CAD build for the part. Positions are in the model's coordinates, mm. A direction names the side the tool comes from. Give positions to 0.01 mm unless a question says otherwise; leave off trailing zeros. Write each loop counter-clockwise with the first axis right and the second up, starting at its lowest first coordinate (ties: lowest second). Pieces come first, ordered by that corner, then holes. Notation, with made-up numbers: (-17.5, 59) -> (-13.5, 59) arc R31 ccw to (-13.5, 86) -> close; hole circle Ø4 at (70, 3). An arc over 180 degrees is marked (long way). Answer as a JSON object with one key per item and string values.
```python
from build123d import *

# Parameters (mm, degrees)
SKETCH002_R                 = 3
EXTRUDE002_DEPTH            = 4
EXTRUDE002_DEPTH_BACK       = 3.4
CYLINDER049_R               = 1.5
CYLINDER049_DEPTH           = 19
CYLINDER014_R               = 2
CYLINDER014_DEPTH           = 1
CYLINDER014_PLACEMENT_ANGLE = 45
CYLINDER015_R               = 2
CYLINDER015_DEPTH           = 1
CYLINDER016_R               = 2
CYLINDER016_DEPTH           = 1
CYLINDER016_PLACEMENT_ANGLE = 135
CYLINDER017_R               = 2
CYLINDER017_DEPTH           = 1
CYLINDER018_R               = 2
CYLINDER018_DEPTH           = 5
CYLINDER018_PLACEMENT_ANGLE = 225
CYLINDER019_R               = 2
CYLINDER019_DEPTH           = 5
CYLINDER020_R               = 2
CYLINDER020_DEPTH           = 5
CYLINDER020_PLACEMENT_ANGLE = 45
CYLINDER013_R               = 2
CYLINDER013_DEPTH           = 1
CYLINDER021_R               = 5
CYLINDER021_DEPTH           = 5
CYLINDER012_R               = 25
CYLINDER012_DEPTH           = 1.5
CUT050_PLACEMENT_ANGLE      = 180


with BuildPart() as extrude002:
    # Sketch002 (on Face25 of Shape005) → Extrude002 (new body, two sides)
    with BuildSketch(Plane(origin=(85.664098, -4.553146, 1.091283), x_dir=(-1, 0, 0), z_dir=(0, 0, 1))) as extrude002_sk:
        with Locations((9.450198, -0.000218)):
            Circle(SKETCH002_R)
    extrude(amount=EXTRUDE002_DEPTH)
    extrude(extrude002_sk.sketch, amount=-EXTRUDE002_DEPTH_BACK)


with BuildPart() as extrude002_1:
    # Extrude002 placement: moved
    add(extrude002.part.moved(Location((-76.21, 4.55, 3))))


with BuildPart() as cylinder049:
    # Cylinder049 → Cylinder049 (new body)
    with BuildSketch(Plane.XY.offset(-1)):
        Circle(CYLINDER049_R)
    extrude(amount=CYLINDER049_DEPTH)


with BuildPart() as cylinder014:
    # cylinder014 → cylinder014 (new body)
    with BuildSketch(Plane.XY):
        Circle(CYLINDER014_R)
    extrude(amount=CYLINDER014_DEPTH)


with BuildPart() as cylinder014_1:
    # cylinder014 placement: moved
    add(cylinder014.part.moved(Location((13.081475, 13.081475, 0))).rotate(Axis((13.081475, 13.081475, 0), (0, 0, 1)), CYLINDER014_PLACEMENT_ANGLE))


with BuildPart() as cylinder015:
    # cylinder015 → cylinder015 (new body)
    with BuildSketch(Plane(origin=(0, 18.5, 0), x_dir=(0, 1, 0), z_dir=(0, 0, 1))):
        Circle(CYLINDER015_R)
    extrude(amount=CYLINDER015_DEPTH)


with BuildPart() as cylinder016:
    # cylinder016 → cylinder016 (new body)
    with BuildSketch(Plane.XY):
        Circle(CYLINDER016_R)
    extrude(amount=CYLINDER016_DEPTH)


with BuildPart() as cylinder016_1:
    # cylinder016 placement: moved
    add(cylinder016.part.moved(Location((-13.081475, 13.081475, 0))).rotate(Axis((-13.081475, 13.081475, 0), (0, 0, 1)), CYLINDER016_PLACEMENT_ANGLE))


with BuildPart() as cylinder017:
    # cylinder017 → cylinder017 (new body)
    with BuildSketch(Plane(origin=(-18.5, 0, 0), x_dir=(-1, 0, 0), z_dir=(0, 0, 1))):
        Circle(CYLINDER017_R)
    extrude(amount=CYLINDER017_DEPTH)


with BuildPart() as cylinder018:
    # cylinder018 → cylinder018 (new body)
    with BuildSketch(Plane.XY):
        Circle(CYLINDER018_R)
    extrude(amount=CYLINDER018_DEPTH)


with BuildPart() as cylinder018_1:
    # cylinder018 placement: moved
    add(cylinder018.part.moved(Location((-13.081475, -13.081475, 0))).rotate(Axis((-13.081475, -13.081475, 0), (0, 0, 1)), CYLINDER018_PLACEMENT_ANGLE))


with BuildPart() as cylinder019:
    # cylinder019 → cylinder019 (new body)
    with BuildSketch(Plane(origin=(0, -18.5, 0), x_dir=(0, -1, 0), z_dir=(0, 0, 1))):
        Circle(CYLINDER019_R)
    extrude(amount=CYLINDER019_DEPTH)


with BuildPart() as cylinder020:
    # cylinder020 → cylinder020 (new body)
    with BuildSketch(Plane.XY):
        Circle(CYLINDER020_R)
    extrude(amount=CYLINDER020_DEPTH)


with BuildPart() as cylinder020_1:
    # cylinder020 placement: moved
    add(cylinder020.part.moved(Location((13.081475, -13.081475, 0))).rotate(Axis((13.081475, -13.081475, 0), (0, 0, -1)), CYLINDER020_PLACEMENT_ANGLE))


with BuildPart() as fusion026:
    # cylinder013 → cylinder013 (new body)
    with BuildSketch(Plane(origin=(18.5, 0, 0), x_dir=(1, 0, 0), z_dir=(0, 0, 1))):
        Circle(CYLINDER013_R)
    extrude(amount=CYLINDER013_DEPTH)

    # Group001: union cylinder014, cylinder015, cylinder016, cylinder017, cylinder018, cylinder019, cylinder020
    add(cylinder014_1.part)
    add(cylinder015.part)
    add(cylinder016_1.part)
    add(cylinder017.part)
    add(cylinder018_1.part)
    add(cylinder019.part)
    add(cylinder020_1.part)


with BuildPart() as fusion026_1:
    # Group001 placement: moved
    add(fusion026.part.moved(Location((0, 0, -1))))

    # Fusion026: union Extrude002, Cylinder049
    add(extrude002_1.part)
    add(cylinder049.part)


with BuildPart() as servo_central_shaft002:
    # cylinder021 → cylinder021 (new body)
    with BuildSketch(Plane.XY):
        Circle(CYLINDER021_R)
    extrude(amount=CYLINDER021_DEPTH)


with BuildPart() as rotor:
    # cylinder012 → cylinder012 (new body)
    with BuildSketch(Plane.XY):
        Circle(CYLINDER012_R)
    extrude(amount=CYLINDER012_DEPTH)

    # Fusion027: union servo_central_shaft002
    add(servo_central_shaft002.part)

    # Cut050: cut Fusion026
    add(fusion026_1.part, mode=Mode.SUBTRACT)


with BuildPart() as rotor_1:
    # Cut050 placement: moved
    add(rotor.part.moved(Location((-13.7, 55.5, 5))).rotate(Axis((-13.7, 55.5, 5), (1, 0, 0)), CUT050_PLACEMENT_ANGLE))


solid = rotor_1.part
```
1) Mould opens along X. For faces 3 (the cylindrical face through (-14.351, 50.543, 1.775)), 4 (the flat face through (-10, 55, 0)), 5 (the cylindrical face through (0.15, 70.43, 4.26)) say: released by +X, released by -X, zero draft, split by the parting line, or undercut.
Model answer:
{"face 3": "split by the parting line", "face 4": "zero draft", "face 5": "undercut"}
2) Slice it at B-B (y = 73). List the corners of the cut face in (x, z).
Model answer:
{"outline": "(-31.55, 3.5) -> (-15.43, 3.5) -> (-15.43, 5) -> (-31.55, 5) -> close; (-11.97, 3.5) -> (4.15, 3.5) -> (4.15, 5) -> (-11.97, 5) -> close"}
3) Slice it at C-C (x = -26.5). List the corners of the cut face in (y, z).
Model answer:
{"outline": "(34.03, 3.5) -> (66.6, 3.5) -> (66.6, 5) -> (34.03, 5) -> close; (70.56, 3.5) -> (76.97, 3.5) -> (76.97, 5) -> (70.56, 5) -> close"}
4) Wall check: probe 1 along Y at (x, z) = (-13.7, 4.15); probe 2 along Z at (x, y) = (0, 42); probe 3 along Y at (x, z) = (-1, 3.9). Give the ranges that are in metal, low to high.
Model answer:
{"probe 1": "y = 30.5 to 52.5, 58.5 to 72, 76 to 80.5", "probe 2": "z = 3.5 to 5", "probe 3": "y = 33.97 to 66.62, 70.54 to 77.03"}
5) Slice it at D-D (z = 1.7). List the corners of the cut face in (x, y).
Model answer:
{"outline": "circle Ø10 at (-13.7, 55.5); hole circle Ø6 at (-13.7, 55.5)"}
6) Pin check, flat tips, straight feed: pin 1 (10 mm diameter, centred on x = -32.5, y = 65, fed in from -Z); pin 2 (3 mm diameter, centred on y = 45.5, z = 0.5, fed in from +X). Stop position of each tip, or through.
Model answer:
{"pin 1": "stops at z = 3.5", "pin 2": "passes through"}
7) 3-axis set-ups, long thin cutter, end or side, ignore diameter. For faces 1 (the flat face through (-8, 55, 5)), 2 (the flat face through (-12, 55, 4.309)): which of +Z, -Z, +X, -X, +Y, -Y reach the whole face in a straight line?
Model answer:
{"face 1": "+Z, +X, -X, +Y, -Y", "face 2": "-Z"}
8) Slice it at A-A (x = -13.7). List the corners of the cut face in (y, z).
Model answer:
{"outline": "(30.5, 3.5) -> (50.5, 3.5) -> (50.5, 0) -> (52.5, 0) -> (52.5, 4.31) -> (54, 4.31) -> (54, 5) -> (30.5, 5) -> close; (57, 4.31) -> (58.5, 4.31) -> (58.5, 0) -> (60.5, 0) -> (60.5, 3.5) -> (72, 3.5) -> (72, 5) -> (57, 5) -> close; (76, 3.5) -> (80.5, 3.5) -> (80.5, 5) -> (76, 5) -> close"}
